Build history of the part. All positions in model axes, mm. A direction names the side the tool comes from. Coordinates: 2 decimals unless noted, no trailing zeros. Order: outer loops, then holes, each group sorted by start corner. A loop starts at its lowest first (then second) coordinate and runs counter-clockwise, first axis right, second up. Notation, with made-up numbers: (13.25, -33.5) - (57.25, -33.5) arc R18 ccw to (57.25, -17.5) - close; hole circle Ø10 at (76, 48.5). An arc over 180 degrees is marked (long way). Return JSON: item names as keys, results as strings.
from build123d import *

# Parameters (mm, degrees)
SKETCH1_W                  = 100
SKETCH1_H                  = 200
BOSS_EXTRUDE1_DEPTH        = 65
F_10_0MM_DOWEL_HOLE1_D     = 10
F_10_0MM_DOWEL_HOLE1_DEPTH = 40
F_10_0MM_DOWEL_HOLE1_TIP   = 3.004303095
SKETCH5_W                  = 50
SKETCH5_H                  = 50
BOSS_EXTRUDE2_DEPTH        = 50


with BuildPart() as part:
    # Sketch1 → Boss-Extrude1 (new body)
    with BuildSketch(Plane(origin=(0, 0, 0), x_dir=(1, 0, 0), z_dir=(0, 1, 0))):
        with Locations((50, 100)):
            Rectangle(SKETCH1_W, SKETCH1_H)
    extrude(amount=BOSS_EXTRUDE1_DEPTH)

    # Ø10.0mm Dowel Hole1
    with Locations(Plane(origin=(0, 65, 0), x_dir=(1, 0, 0), z_dir=(0, 1, 0))):
        with Locations((50, 100)):
            Hole(F_10_0MM_DOWEL_HOLE1_D / 2, depth=F_10_0MM_DOWEL_HOLE1_DEPTH)
            with Locations((0, 0, -(F_10_0MM_DOWEL_HOLE1_DEPTH + F_10_0MM_DOWEL_HOLE1_TIP / 2))):  # 118° drill point
                Cone(0, F_10_0MM_DOWEL_HOLE1_D / 2, F_10_0MM_DOWEL_HOLE1_TIP, mode=Mode.SUBTRACT)

    # Sketch5 → Boss-Extrude2 (add)
    with BuildSketch(Plane(origin=(0, 65, 0), x_dir=(1, 0, 0), z_dir=(0, 1, 0))):
        with Locations((25, 25)):
            Rectangle(SKETCH5_W, SKETCH5_H)
    extrude(amount=BOSS_EXTRUDE2_DEPTH)


solid = part.part
1. Tool access for faces 1 (the flat face through (49, 32, -200)), 2 (the flat face through (25, 90, -50)), 3 (the flat face through (50, 90, -25)): list every direction of +Z, -Z, +X, -X, +Y, -Y with a clear straight run to the whole face (end or side of a thin tool).
Check values:
{"face 1": "-Z, +X, -X, +Y, -Y", "face 2": "-Z, +X, -X, +Y", "face 3": "+Z, -Z, +X, +Y"}
2. Probe L1, parallel to X at y = 43, z = -100; L2, parallel to Z at x = 50, y = 43; L3, parallel to Y at x = 84.5, z = -26.5. List the from-to ranges inside material, lowest first.
Check values:
{"L1": "0 to 45, 55 to 100", "L2": "-200 to -105, -95 to 0", "L3": "0 to 65"}
3. Drop flat-ended pins along their axis: pin 1 (4 mm diameter, centred on x = 74, z = -117.5, fed in from +Y); pin 2 (15 mm diameter, centred on x = 28, y = 83.5, fed in from -Z); pin 3 (15 mm diameter, centred on y = 93, z = -24.5, fed in from +X). Give the stop position or say it passes through.
Check values:
{"pin 1": "y = 65", "pin 2": "z = -50", "pin 3": "x = 50"}
4. Cut at C-C on y = 106. Give the cut face in (x, z).
Check values:
{"outline": "(0, -50) - (50, -50) - (50, 0) - (0, 0) - close"}
5. Mould opens along X. For faces 4 (the flat face through (49, 0, -101)), 5 (the flat face through (0, 44, -76)), 6 (the cylindrical face through (54, 45, -103)) say: pulls with the +X half, pulls with the -X half, needs draft (parallel to the pull), parting line crosses it, or undercut.
Check values:
{"face 4": "needs draft", "face 5": "pulls with the -X half", "face 6": "undercut"}
6. Cut at B-B on z = -140. Give the cut face in (x, y).
Check values:
{"outline": "(0, 0) - (100, 0) - (100, 65) - (0, 65) - close"}
7. Cut at A-A on x = 17. Give the cut face in (y, z), plus the area to 3 significant figures.
Check values:
{"outline": "(0, -200) - (65, -200) - (65, -50) - (115, -50) - (115, 0) - (0, 0) - close", "area": "15,500 mm²"}
